Geometry: final body of the model. Coordinates: model frame, mm. A direction names the side the tool comes from. Coordinates: 2 decimals unless noted, no trailing zeros. Loops run counter-clockwise (first coordinate to the right, second up) from the corner with the lowest first, then second, coordinate; pieces in that order, holes last. Notation, with made-up numbers: M 28,45 L 77,45 A33 cw 77,79 Z; hole C 41.5,75.5 d3. An arc over 180 degrees is marked long. Write item = value, one per line. Start each with the question number.
```python
from build123d import *

# Parameters (mm, degrees)
F1_DEPTH = 1.27
F0_W     = 1.27
F0_H     = 25.4


with BuildPart() as f1:
    # F0 (on Front) → F1 (new body, symmetric)
    with BuildSketch(Plane.XZ):
        Polygon((-38.1, 27.94), (-38.1, 25.4), (-36.83, 25.4), (36.83, 25.4), (38.1, 25.4), (38.1, 27.94), align=None)
    extrude(amount=F1_DEPTH, both=True)

    # F0 (on Front) → F2 (revolve)
    with BuildSketch(Plane.XZ):
        with Locations((-37.465, 12.7)):
            Rectangle(F0_W, F0_H)
    revolve(axis=Axis((-36.83, 0, 12.7), (0, 0, 1)))

    # F0 (on Front) → F3 (revolve)
    with BuildSketch(Plane.XZ):
        with Locations((37.465, 12.7)):
            Rectangle(F0_W, F0_H)
    revolve(axis=Axis((36.83, 0, 12.7), (0, 0, 1)))


solid = f1.part
```
Item 1: Section query C-C (x = -33). Return the cut outline in (y, z).
Item 2: Line query: line 1 (X direction, y = 0.1, z = 13.5); line 2 (Z direction, x = 3.5, y = -0.3); line 3 (X direction, y = -0.75, z = 14.5). Output: solid intervals per line, ascending. Write a range as from..to.
Item 3: Reachability of faces 1 (the flat face through (37.8, -1.1, 25.4)), 2 (the flat face through (37.84, 1.01, 25.4)), 3 (the flat face through (-37.84, 1.01, 25.4)), 4 (the flat face through (37, 0, 0)), 5 (the flat face through (-1, 1.27, 27)) from +Z, -Z, +X, -X, +Y, -Y: full face, straight path, thin tool, end or side. Return the list, or none.
Item 4: Section query B-B (y = 0.75). Return the cut outline in (x, z), plus the area to 3 significant figures.
Item 5: Section query A-A (z = 18.25). Return the cut outline in (x, y), plus the area to 3 significant figures.
Item 6: Pull-direction query (X, two-part tool) for faces 6 (the flat face through (-38.1, 0, 27)), 7 (the flat face through (-37.9, -1, 25.4)), 8 (the cylindrical face through (35.82, -0.77, 12.88)), 9 (the cylindrical face through (-35.82, 0.77, 12.88)); classes: released by +X, released by -X, zero draft, split by the parting line, or undercut.
Verdict:
q1.outline = M -1.27,25.4 L 1.27,25.4 L 1.27,27.94 L -1.27,27.94 Z
q2.line_1 = -38.1..-35.56, 35.56..38.1
q2.line_2 = 25.4..27.94
q2.line_3 = -37.85..-35.81, 35.81..37.85
q3.face_1 = -Z, +X, -Y
q3.face_2 = -Z, +X, +Y
q3.face_3 = -Z, -X, +Y
q3.face_4 = -Z, +X, -X, +Y, -Y
q3.face_5 = +Z, -Z, +X, -X, +Y
q4.outline = M -38.1,25.4 L -37.85,25.4 L -37.85,0 L -35.81,0 L -35.81,25.4 L 35.81,25.4 L 35.81,0 L 37.85,0 L 37.85,25.4 L 38.1,25.4 L 38.1,27.94 L -38.1,27.94 Z
q4.area = 298 mm2
q5.outline = C -36.83,0 d2.54; C 36.83,0 d2.54
q5.area = 10.1 mm2
q6.face_6 = released by -X
q6.face_7 = zero draft
q6.face_8 = undercut
q6.face_9 = undercut
